The drawing under review shows one solid part. Ordinate dimensions are in mm from its lowest x, y, z. Round coordinates to 2 decimals unless told otherwise and drop trailing zeros. Write each loop counter-clockwise with the first axis right and the second up, starting at its lowest first coordinate (ties: lowest second). Pieces come first, ordered by that corner, then holes. Notation, with made-up numbers: M -25,33.25 L 7,33.25 A16 cw 7,42.25 Z; hole C -37,76.5 d3. An arc over 180 degrees is marked long. Write item = value, one per line. Start each with the question number.
Item 1: Take a section at B-B, the plane y = 31. Give the boundary of the cut face in (x, z).
Item 2: For pin 1 Ø1 at (x, z) = (26.5, 28) entering from -Y, flat-tipped, find the tip position at first contact; note if it passes through.
Item 3: Take a section at A-A, the plane x = 28. Give the boundary of the cut face in (y, z).
Item 4: To check wall thickness, follow line 1 along Y through (x, z) = (26.5, 25); line 2 along X through (y, z) = (24.5, 25) (1 decimal); line 3 along X through (y, z) = (24, 23.5) (1 decimal). State the ranges of each line that lie inside material, in increasing order.
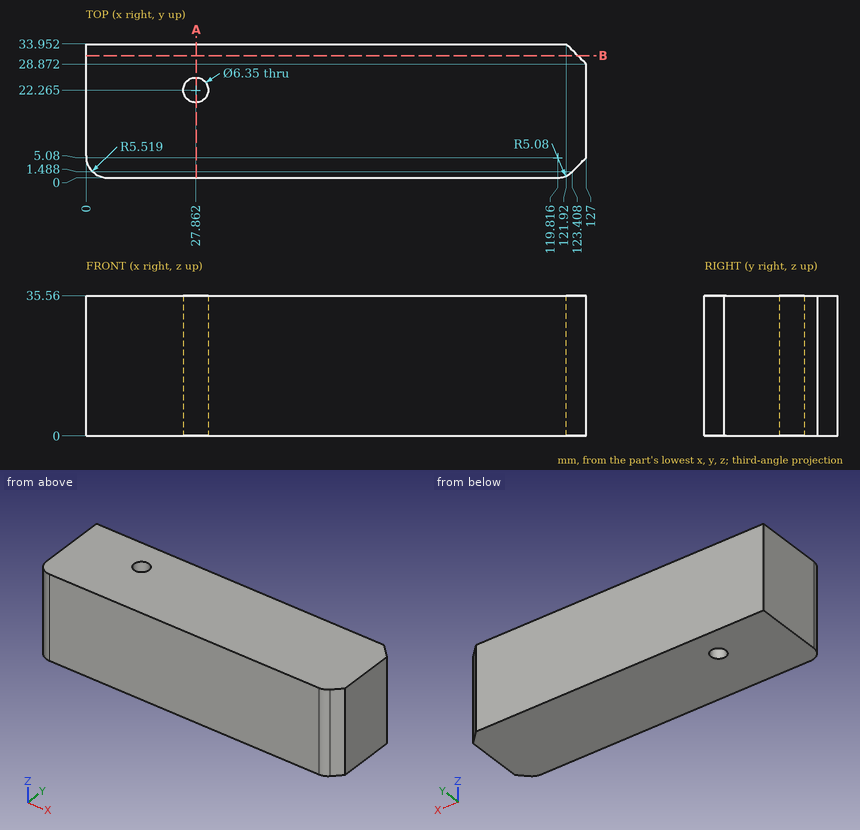
Response values:
q1.outline = M 0,0 L 124.87,0 L 124.87,35.56 L 0,35.56 Z
q2.pin_1 = 0
q3.outline = M 0,0 L 19.09,0 L 19.09,35.56 L 0,35.56 Z; M 25.44,0 L 33.95,0 L 33.95,35.56 L 25.44,35.56 Z
q4.line_1 = 0 to 19.4, 25.13 to 33.95
q4.line_2 = 0 to 25.6, 30.1 to 127
q4.line_3 = 0 to 25.2, 30.5 to 127
